The model under review builds one solid part; all positions refer to its coordinate system, in mm. Face numbers are marked on the shaded views. Give positions to 0.01 mm unless a question says otherwise; leave off trailing zeros. Write each loop counter-clockwise with the first axis right and the second up, starting at its lowest first coordinate (ties: lowest second). Pieces come first, ordered by that corner, then holes. Notation, with made-up numbers: (-5, -24) -> (11, -24) arc R17 cw to (11, -3) -> close; hole circle Ø6 at (33.5, 56.25). An arc over 180 degrees is marked (long way). Use CSV: the item, a comma, the result in double quotes.
```python
from build123d import *

# Parameters (mm, degrees)
F1_DEPTH = 3.25
F3_DEPTH = 2.5
F5_DEPTH = 3


with BuildPart() as f1:
    # F0 (on Right) → F1 (new body)
    with BuildSketch(Plane.YZ):
        with BuildLine():
            Line((-12.5, 0), (-12.5, -3))
            Line((-12.5, -3), (12.5, -3))
            Line((12.5, -3), (12.5, 0))
            Line((12.5, 0), (4.5, 0))
            ThreePointArc((4.5, 0), (0, -1.5), (-4.5, 0))
            Line((-4.5, 0), (-12.5, 0))
        make_face()
    extrude(amount=F1_DEPTH)

    # F2 (on face) → F3 (join)
    with BuildSketch(Plane.YZ.offset(3.25)):
        with BuildLine():
            Line((-2.624389, 9.655486), (-4.5, 8.308926))
            Line((-4.5, 8.308926), (-10.415988, 4.061652))
            ThreePointArc((-10.415988, 4.061652), (-11.948592, 2.282549), (-12.5, 0))
            Line((-12.5, 0), (-12.5, -3))
            Line((-12.5, -3), (12.5, -3))
            Line((12.5, -3), (12.5, 0))
            ThreePointArc((12.5, 0), (11.948592, 2.282549), (10.415988, 4.061652))
            Line((10.415988, 4.061652), (4.5, 8.308926))
            Line((4.5, 8.308926), (2.624389, 9.655486))
            ThreePointArc((2.624389, 9.655486), (0, 10.5), (-2.624389, 9.655486))
        make_face()
        with BuildLine():
            ThreePointArc((2, 6), (0, 4), (-2, 6))
            ThreePointArc((-2, 6), (0, 8), (2, 6))
        make_face(mode=Mode.SUBTRACT)
    extrude(amount=F3_DEPTH)

    # F4 (on face) → F5 (join, through all)
    with BuildSketch(Plane(origin=(0, 0, -3), x_dir=(1, 0, 0), z_dir=(0, 0, -1))):
        Polygon((4.75, -11.5), (0, -11.5), (0, -22.5), (10.75, -22.5), (15.75, -17.5), (15.75, 17.5), (10.75, 22.5), (0, 22.5), (0, 11.5), (4.75, 11.5), align=None)
    extrude(amount=-F5_DEPTH)

    # F6: F1 across plane


with BuildPart() as f1_1:
    add(f1.part)
    add(f1.part.mirror(Plane.YZ))


solid = f1_1.part
```
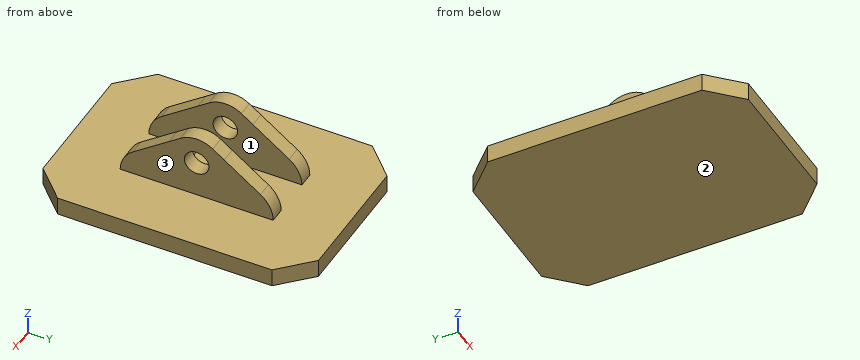
Q1. Consider section D-D (z = 0.75). Write out the cut boundary in (x, y).
Derived:
outline,"(-5.75, -12.44) -> (-3.25, -12.44) -> (-3.25, 12.44) -> (-5.75, 12.44) -> close; (3.25, -12.44) -> (5.75, -12.44) -> (5.75, 12.44) -> (3.25, 12.44) -> close"
Q2. To check wall thickness, follow probe 1 along Z at (x, y) = (-4, 0); probe 2 along X at (y, z) = (2, 0.5); probe 3 along Z at (x, y) = (11, -17). State the ranges of each line that lie inside material, in increasing order.
Derived:
probe 1,"z = -3 to 4, 8 to 10.5"
probe 2,"x = -5.75 to -3.25, 3.25 to 5.75"
probe 3,"z = -3 to 0"
Q3. Consider section A-A (y = 0). Write out the cut boundary in (x, z), then the cut area to 3 significant figures.
Derived:
outline,"(-15.75, -3) -> (15.75, -3) -> (15.75, 0) -> (5.75, 0) -> (5.75, 4) -> (3.25, 4) -> (3.25, -1.5) -> (-3.25, -1.5) -> (-3.25, 4) -> (-5.75, 4) -> (-5.75, 0) -> (-15.75, 0) -> close; (-5.75, 8) -> (-3.25, 8) -> (-3.25, 10.5) -> (-5.75, 10.5) -> close; (3.25, 8) -> (5.75, 8) -> (5.75, 10.5) -> (3.25, 10.5) -> close"
area,"117 mm2"
Q4. Insertion check: pin 1 (4 mm diameter, centred on y = 2.5, z = 5.5, fed in from +X); pin 2 (2 mm diameter, centred on x = -3.5, z = 6, fed in from +Y); pin 3 (6.5 mm diameter, centred on y = 0, z = 6, fed in from -X). Each pin has a flat end and moves straight along its axis. Give the tip position at first contact, or say it passes through.
Derived:
pin 1,"stops at x = 5.75"
pin 2,"stops at y = 9.11"
pin 3,"stops at x = -5.75"
Q5. Consider section B-B (z = 7.25). Write out the cut boundary in (x, y).
Derived:
outline,"(-5.75, -5.97) -> (-3.25, -5.97) -> (-3.25, -1.56) -> (-5.75, -1.56) -> close; (-5.75, 1.56) -> (-3.25, 1.56) -> (-3.25, 5.97) -> (-5.75, 5.97) -> close; (3.25, -5.97) -> (5.75, -5.97) -> (5.75, -1.56) -> (3.25, -1.56) -> close; (3.25, 1.56) -> (5.75, 1.56) -> (5.75, 5.97) -> (3.25, 5.97) -> close"
Q6. The part is to be moulded in two halves that separate along X. For the marked faces 1, 2 and 3, say which applies: pulls with the +X half, pulls with the -X half, needs draft (parallel to the pull), parting line crosses it, or undercut.
Derived:
face 1,"undercut"
face 2,"needs draft"
face 3,"pulls with the +X half"
Q7. Consider section C-C (x = 1.5). Write out the cut boundary in (y, z), then the cut area to 3 significant figures.
Derived:
outline,"(-22.5, -3) -> (22.5, -3) -> (22.5, 0) -> (4.5, 0) arc R7.5 cw to (-4.5, 0) -> (-22.5, 0) -> close"
area,"126 mm2"
